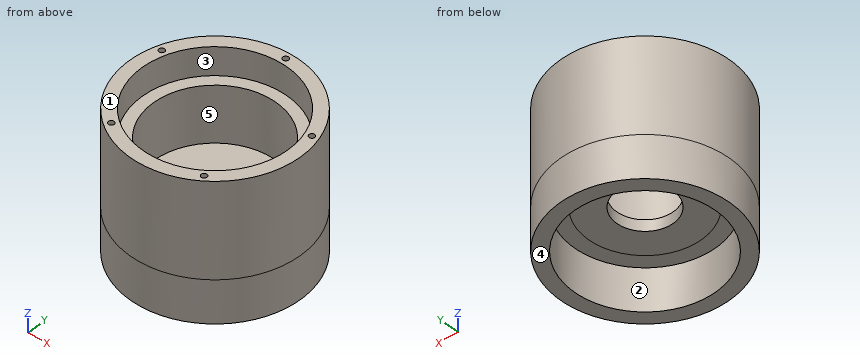
```python
from build123d import *

# Parameters (mm, degrees)
SKETCH2_R           = 76.2
BOSS_EXTRUDE1_DEPTH = 85
SKETCH4_R           = 65
CUT_EXTRUDE2_DEPTH  = 25
SKETCH5_R           = 55
CUT_EXTRUDE3_DEPTH  = 50
SKETCH7_R           = 2.5
CUT_EXTRUDE4_DEPTH  = 20
CIRPATTERN1_COUNT   = 5
BOSS_EXTRUDE2_START = 38.1
SKETCH8_R           = 76.2
SKETCH8_R_2         = 50.8
BOSS_EXTRUDE2_DEPTH = 38.1


with BuildPart() as part:
    # Sketch2 → Boss-Extrude1 (new body)
    with BuildSketch(Plane(origin=(0, 0, 0), x_dir=(0, 1, 0), z_dir=(0, 0, 1))):
        with Locations(Location((0, 0, 0), (0, 0, 270))):
            Circle(SKETCH2_R)
    extrude(amount=BOSS_EXTRUDE1_DEPTH)

    # Sketch4 → Cut-Extrude2 (cut)
    with BuildSketch(Plane.XY.offset(85)):
        Circle(SKETCH4_R)
    extrude(amount=-CUT_EXTRUDE2_DEPTH, mode=Mode.SUBTRACT)

    # Sketch5 → Cut-Extrude3 (cut)
    with BuildSketch(Plane.XY.offset(60)):
        Circle(SKETCH5_R)
    extrude(amount=-CUT_EXTRUDE3_DEPTH, mode=Mode.SUBTRACT)

    # Sketch7 → Cut-Extrude4 (cut)
    with BuildSketch(Plane.XY.offset(85)):
        with Locations((0, 70.612)):
            Circle(SKETCH7_R)
    cut_extrude4 = extrude(amount=-CUT_EXTRUDE4_DEPTH, mode=Mode.SUBTRACT)

    # CirPattern1: Cut-Extrude4 ×5 about axis
    cirpattern1_axis = Axis((0, 0, 0), (0, 0, 1))
    for i in range(1, CIRPATTERN1_COUNT):
        add(cut_extrude4.rotate(cirpattern1_axis, i * 360 / CIRPATTERN1_COUNT), mode=Mode.SUBTRACT)

    # Sketch8 → Boss-Extrude2 (add)
    with BuildSketch(Plane(origin=(0, 0, 0), x_dir=(1, 0, 0), z_dir=(0, 0, -1)).offset(BOSS_EXTRUDE2_START)):
        with Locations(Location((0, 0, 0), (0, 0, 180))):
            Circle(SKETCH8_R)
        Circle(SKETCH8_R_2, mode=Mode.SUBTRACT)
    extrude(amount=-BOSS_EXTRUDE2_DEPTH)

    # Sketch10 → Cut-Revolve1 (revolve, cut)
    with BuildSketch(Plane.YZ, mode=Mode.PRIVATE) as cut_revolve1_sk:
        Polygon((0, 10.519966747), (-25.372140722, 10), (-25.372140722, 0), (-63.592993734, 0), (-63.592993734, -38.1), (0, -38.1), align=None)
    revolve(cut_revolve1_sk.sketch.rotate(Axis((0, 0, -38.1), (0, 0, 1)), 270), axis=Axis((0, 0, -38.1), (0, 0, 1)), mode=Mode.SUBTRACT)


solid = part.part
```
Verification items for the finished model (mm, model axes). Face numbers are marked on the shaded views. A direction names the side the tool comes from. Round coordinates to 2 decimals unless told otherwise and drop trailing zeros. Loops run counter-clockwise (first coordinate to the right, second up) from the corner with the lowest first, then second, coordinate; pieces in that order, holes last. Notation, with made-up numbers: (47.5, 58) -> (52.5, 58) arc R33 ccw to (52.5, 91) -> close; hole circle Ø4 at (34, 13). An arc over 180 degrees is marked (long way). Answer as a JSON object with one key per item and string values.
Q1. Section check C-C (z = 21.5). Record the boundary of the cut face in (x, y), then the cut area to 3 significant figures.
Data:
{"outline": "circle Ø152.4 at (0, 0); hole circle Ø110 at (0, 0)", "area": "8,740 mm2"}
Q2. Section check B-B (x = 0). Record the boundary of the cut face in (y, z), then the cut area to 3 significant figures.
Data:
{"outline": "(-76.2, -38.1) -> (-63.59, -38.1) -> (-63.59, 0) -> (-25.37, 0) -> (-25.37, 10) -> (-55, 10) -> (-55, 60) -> (-65, 60) -> (-65, 85) -> (-76.2, 85) -> close; (25.37, 0) -> (63.59, 0) -> (63.59, -38.1) -> (76.2, -38.1) -> (76.2, 85) -> (73.11, 85) -> (73.11, 65) -> (68.11, 65) -> (68.11, 85) -> (65, 85) -> (65, 60) -> (55, 60) -> (55, 10) -> (25.37, 10) -> close", "area": "4,560 mm2"}
Q3. Access from +Z, -Z, +X, -X, +Y, -Y to the whole of each face (thin tool, end or side, straight path). Record for the marked faces 1, 2 and 3.
Data:
{"face 1": "+Z, +X, -X, +Y, -Y", "face 2": "-Z", "face 3": "+Z"}
Q4. Go/stop test with flat-tipped pins: P1, Ø5, axis at x = -27.5, y = -17, coming from the +Z side; P2, Ø3, axis at x = -67.16, y = 21.82, coming from the +Z side; P3, Ø1.5, axis at x = -33.5, z = 32.5, coming from the -Y side. Record where each tip stops, or that it passes through.
Data:
{"P1": "stops at z = 10", "P2": "stops at z = 65", "P3": "stops at y = -68.8"}
Q5. Section check A-A (y = 0). Record the boundary of the cut face in (x, z).
Data:
{"outline": "(-76.2, -38.1) -> (-63.59, -38.1) -> (-63.59, 0) -> (-25.37, 0) -> (-25.37, 10) -> (-55, 10) -> (-55, 60) -> (-65, 60) -> (-65, 85) -> (-76.2, 85) -> close; (25.37, 0) -> (63.59, 0) -> (63.59, -38.1) -> (76.2, -38.1) -> (76.2, 85) -> (65, 85) -> (65, 60) -> (55, 60) -> (55, 10) -> (25.37, 10) -> close"}
Q6. Scan lines: line 1 (Y direction, x = 0, z = 69.25); line 2 (Y direction, x = 0, z = 5.75); line 3 (Z direction, x = -9, y = 46.5). Record each from-to range of solid material in increasing order. Write a range as from..to.
Data:
{"line 1": "y = -76.2..-65, 65..68.11, 73.11..76.2", "line 2": "y = -76.2..-25.37, 25.37..76.2", "line 3": "z = 0..10"}
Q7. Draft check along Y on the marked faces 4 and 5. Enter one of: pulls with the +Y half, pulls with the -Y half, needs draft (parallel to the pull), parting line crosses it, or undercut.
Data:
{"face 4": "needs draft", "face 5": "undercut"}
Q8. Section check D-D (x = -58.5). Record the boundary of the cut face in (y, z).
Data:
{"outline": "(-48.83, -38.1) -> (-24.94, -38.1) -> (-24.94, 0) -> (24.94, 0) -> (24.94, -38.1) -> (48.83, -38.1) -> (48.83, 85) -> (28.33, 85) -> (28.33, 60) -> (-28.33, 60) -> (-28.33, 85) -> (-48.83, 85) -> close"}
